```python
from build123d import *

# Parameters (mm, degrees)
BOSS_EXTRUDE1_DEPTH = 20
CUT_EXTRUDE1_START  = -2.5
SKETCH2_R           = 12
SKETCH2_R_2         = 4
CUT_EXTRUDE1_DEPTH  = 15
FILLET1_R           = 2
BOSS_EXTRUDE2_DEPTH = 20


with BuildPart() as part:
    # Sketch1 → Boss-Extrude1 (new body)
    with BuildSketch(Plane(origin=(0, 0, 0), x_dir=(0, 0, -1), z_dir=(1, 0, 0))):
        with BuildLine():
            Line((0, 0), (-40, 0))
            ThreePointArc((-40, 0), (-62.908712115, -5), (-40, -10))
            Line((-40, -10), (0, -10))
            Line((0, -10), (0, 0))
        make_face()
    extrude(amount=BOSS_EXTRUDE1_DEPTH)

    # Sketch2 → Cut-Extrude1 (cut)
    with BuildSketch(Plane(origin=(20, 0, 0), x_dir=(0, 0, -1), z_dir=(1, 0, 0)).offset(CUT_EXTRUDE1_START)):
        with Locations((-50.908712115, -5)):
            Circle(SKETCH2_R)
        with Locations((-50.908712115, -5)):
            Circle(SKETCH2_R_2, mode=Mode.SUBTRACT)
    extrude(amount=-CUT_EXTRUDE1_DEPTH, mode=Mode.SUBTRACT)

    # Fillet1
    fillet1_edges = [part.edges().sort_by_distance(p)[0] for p in [
        (0, -5, 62.908712115),
        (20, -5, 62.908712115),
        (10, -10, 40),
        (10, 0, 40),
    ]]
    fillet(fillet1_edges, radius=FILLET1_R)

    # Sketch3 → Boss-Extrude2 (add)
    with BuildSketch(Plane(origin=(20, 0, 0), x_dir=(0, 0, -1), z_dir=(1, 0, 0))):
        with BuildLine():
            Line((0, 0), (29.54423259, -5.20944533))
            Line((29.54423259, -5.20944533), (52.525565884, -24.493073621))
            ThreePointArc((52.525565884, -24.493073621), (52.883353103, -28.709461138), (48.668892888, -29.089277519))
            Line((48.668892888, -29.089277519), (30, -15.289809421))
            Line((30, -15.289809421), (0, -10))
            Line((0, -10), (0, 0))
        make_face()
    extrude(amount=-BOSS_EXTRUDE2_DEPTH)


solid = part.part
```
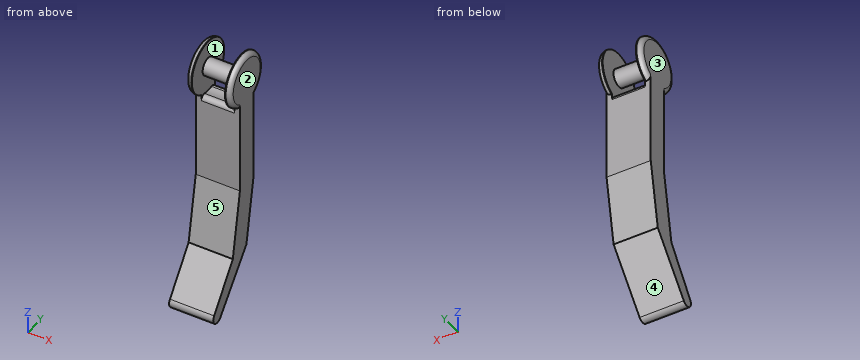
Here's how the part is built. I have some questions about the finished solid (model axes, mm). Face numbers are marked on the shaded views. A direction names the side the tool comes from. Coordinates: 2 decimals unless noted, no trailing zeros. Write each loop counter-clockwise with the first axis right and the second up, starting at its lowest first coordinate (ties: lowest second). Pieces come first, ordered by that corner, then holes. Notation, with made-up numbers: (62.5, 87) -> (83.5, 87) arc R28 ccw to (83.5, 117) -> close; hole circle Ø3 at (32.5, 28). An arc over 180 degrees is marked (long way). Use a Markdown table: item, result. Add a question column.
(1) For the marked faces 1 and 2, which set-ups out of +Z, -Z, +X, -X, +Y, -Y let a thin tool reach every point of the face, with its end or its side?
(2) We'd pull the mould along Z, two halves only. Please class the marked faces 3, 4 and 5: +Z half, -Z half, draft (parallel to the pull), parting line (faces both ways), or undercut.
(3) I'm going to push flat-ended pins straight in: P1, Ø4, axis at x = 17.5, z = -13.5, coming from the +Y side; P2, Ø6, axis at x = 5, z = 22, coming from the -Y side; P3, Ø1, axis at x = 8, z = -21.5, coming from the -Y side; P4, Ø7, axis at y = -3, z = 50.5, coming from the -X side. Where does each tip first touch, or does it pass through?
(4) If we section it at C-C, the plane z = -22: Write out the boundary of the cut face in (x, y), and give its area (3 significant figures).
(5) Please list where these lines run through material, in increasing order: line 1 (Y direction, x = 14, z = 14); line 2 (Z direction, x = 11.5, y = -23.5); line 3 (Z direction, x = 5, y = -7).
(6) If we section it at A-A, the plane x = 8.25: Write out the boundary of the cut face in (y, z).
(7) If we section it at B-B, the plane y = -19: Write out the boundary of the cut face in (x, z).
Outcome:
| question | item | result |
|---|---|---|
| 1 | face 1 | none |
| 1 | face 2 | +Z, -Z, +X, +Y, -Y |
| 2 | face 3 | draft |
| 2 | face 4 | -Z half |
| 2 | face 5 | undercut |
| 3 | P1 | stops at y = -2.03 |
| 3 | P2 | stops at y = -10 |
| 3 | P3 | stops at y = -13.88 |
| 3 | P4 | stops at x = 0 |
| 4 | outline | (0, -13.88) -> (20, -13.88) -> (20, -3.88) -> (0, -3.88) -> close |
| 4 | area | 200 mm^2 |
| 5 | line 1 | y = -10 to 0 |
| 5 | line 2 | z = -51.34 to -41.11 |
| 5 | line 3 | z = -31.68 to 39.08, 47.44 to 54.37 |
| 6 | outline | (-29.09, -48.67) arc R3 ccw to (-24.49, -52.53) -> (-5.21, -29.54) -> (0, 0) -> (0, 37.23) arc R2 ccw to (-2.43, 39.19) arc R12 cw to (-7.57, 39.19) arc R2 ccw to (-10, 37.23) -> (-10, 0) -> (-15.29, -30) -> close; circle Ø8 at (-5, 50.91) |
| 7 | outline | (0, -45.98) -> (20, -45.98) -> (20, -35.02) -> (0, -35.02) -> close |
